Design review of the part built by this model. Coordinates are the model's own, in mm. Round coordinates to 2 decimals unless told otherwise and drop trailing zeros. Order: outer loops, then holes, each group sorted by start corner. A loop starts at its lowest first (then second) coordinate and runs counter-clockwise, first axis right, second up. Notation, with made-up numbers: M -9,-7 L 9,-7 A17 cw 9,7 Z; hole C 15.25,-4.75 d6. An arc over 180 degrees is marked long. Write each question's results on one line, items separated by ' | '. Start each with the question number.
Item 1: Wall thickness on line 1 (Y direction, x = 82.05, z = -3); line 2 (Z direction, x = 29.5, y = -16.5); line 3 (X direction, y = -26, z = -4): over which ranges is each line inside the solid? List them lowest first. Write a range as [from, to].
Item 2: Clearance check with flat-ended pins moving along their axes: pin 1 (6.5 mm diameter, centred on y = 0.5, z = -4, fed in from +X); pin 2 (3 mm diameter, centred on x = -39, y = -13, fed in from -Z); pin 3 (5 mm diameter, centred on x = -81, z = -5.5, fed in from -Y); pin 4 (1.2 mm diameter, centred on y = 5, z = 2.5, fed in from +X). State where each tip first meets the part, or that it passes through.
Item 3: Take a section at B-B, the plane x = 38. Write out the cut boundary in (y, z).
Item 4: Take a section at A-A, the plane y = 0. Write out the cut boundary in (x, z), plus the area to 3 significant figures.
Item 5: Take a section at C-C, the plane y = 8. Write out the cut boundary in (x, z), plus the area to 3 significant figures.
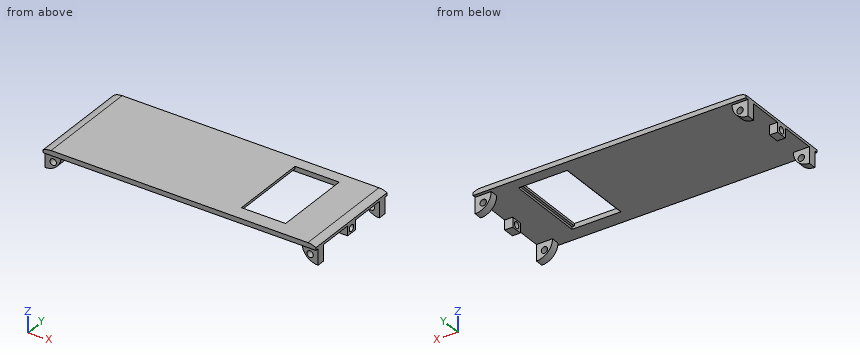
```python
from build123d import *

# Parameters (mm, degrees)
SKIZZE1_W                                  = 180
SKIZZE1_H                                  = 65
AUFSATZ_LINEAR_AUSTRAGEN1_DEPTH            = 3
SKIZZE3_W                                  = 5
SKIZZE3_H                                  = 7
AUFSATZ_LINEAR_AUSTRAGEN2_DEPTH            = 6
F_4_0_4_DURCHMESSER_BOHRUNG1_D             = 4
SCHNITT_LINEAR_AUSTRAGEN1_DEPTH            = 112.180034179
SKIZZE7_W                                  = 27.5
SKIZZE7_H                                  = 49
SCHNITT_LINEAR_AUSTRAGEN2_DEPTH            = 92.445338864
SKIZZE8_W                                  = 10
SKIZZE8_H                                  = 5
AUFSATZ_LINEAR_AUSTRAGEN3_DEPTH            = 10
SPIEGELN1_AT_THE_SECOND_PLANE_COPY_1_SKE_W = 10
SPIEGELN1_AT_THE_SECOND_PLANE_COPY_1_SKE_H = 5
SPIEGELN1_AT_THE_SECOND_PLANE_COPY_1_DEPTH = 10
VERRUNDUNG1_R                              = 10
F_4_0_4_DURCHMESSER_BOHRUNG2_D             = 4
F_4_0_4_DURCHMESSER_BOHRUNG2_DEPTH         = 5
F_4_0_4_DURCHMESSER_BOHRUNG3_D             = 4
F_4_0_4_DURCHMESSER_BOHRUNG3_DEPTH         = 5
SKIZZE13_W                                 = 30.5
SKIZZE13_H                                 = 49
SCHNITT_LINEAR_AUSTRAGEN4_DEPTH            = 1.5


with BuildPart() as part:
    # Skizze1 → Aufsatz-Linear austragen1 (new body)
    with BuildSketch(Plane.XY):
        Rectangle(SKIZZE1_W, SKIZZE1_H)
    extrude(amount=AUFSATZ_LINEAR_AUSTRAGEN1_DEPTH)

    # Skizze3 → Aufsatz-Linear austragen2 (add)
    with BuildSketch(Plane(origin=(0, 0, 0), x_dir=(-1, 0, 0), z_dir=(0, 0, -1))):
        with Locations((-82.5, 0)):
            Rectangle(SKIZZE3_W, SKIZZE3_H)
        with Locations((82.5, 0)):
            Rectangle(SKIZZE3_W, SKIZZE3_H)
    extrude(amount=AUFSATZ_LINEAR_AUSTRAGEN2_DEPTH)

    # Ø4.0 (4) Durchmesser Bohrung1 (through all)
    with Locations(Plane.ZY.offset(85)):
        with Locations((-3, 0)):
            Hole(F_4_0_4_DURCHMESSER_BOHRUNG1_D / 2)

    # Skizze6 → Schnitt-Linear austragen1 (cut, through all)
    with BuildSketch(Plane(origin=(0, 32.5, 0), x_dir=(1, 0, 0), z_dir=(0, 1, 0))):
        with BuildLine():
            Line((-80, -3), (-90, -3))
            Line((-90, -3), (-90, 0))
            Line((-90, 0), (-85, 0))
            Line((-85, 0), (-85, -1.660254038))
            ThreePointArc((-85, -1.660254038), (-82.588190451, -2.659258263), (-80, -3))
        make_face()
        with BuildLine():
            Line((80, -3), (90, -3))
            Line((90, -3), (90, 0))
            Line((90, 0), (85, 0))
            Line((85, 0), (85, -1.660254038))
            ThreePointArc((85, -1.660254038), (82.588190451, -2.659258263), (80, -3))
        make_face()
    extrude(amount=-SCHNITT_LINEAR_AUSTRAGEN1_DEPTH, mode=Mode.SUBTRACT)

    # Skizze7 → Schnitt-Linear austragen2 (cut, through all)
    with BuildSketch(Plane.XY.offset(3)):
        with Locations((46.25, 1)):
            Rectangle(SKIZZE7_W, SKIZZE7_H)
    extrude(amount=-SCHNITT_LINEAR_AUSTRAGEN2_DEPTH, mode=Mode.SUBTRACT)

    # Skizze8 → Aufsatz-Linear austragen3 (add)
    with BuildSketch(Plane(origin=(0, 0, 0), x_dir=(-1, 0, 0), z_dir=(0, 0, -1))):
        with Locations((-80, 28)):
            Rectangle(SKIZZE8_W, SKIZZE8_H)
    aufsatz_linear_austragen3 = extrude(amount=AUFSATZ_LINEAR_AUSTRAGEN3_DEPTH)

    # Spiegeln1: Aufsatz-Linear austragen3 across plane
    add(aufsatz_linear_austragen3.mirror(Plane(origin=(0, 0, 0), x_dir=(0, 0, 1), z_dir=(1, 0, 0))))

    # Spiegeln1 at the second plane: Aufsatz-Linear austragen3 across plane
    add(aufsatz_linear_austragen3.mirror(Plane.ZX))

    # Spiegeln1 at the second plane copy 1 ske → Spiegeln1 at the second plane copy 1 (add)
    with BuildSketch(Plane(origin=(0, 0, 0), x_dir=(1, 0, 0), z_dir=(0, 0, -1))):
        with Locations((-80, 28)):
            Rectangle(SPIEGELN1_AT_THE_SECOND_PLANE_COPY_1_SKE_W, SPIEGELN1_AT_THE_SECOND_PLANE_COPY_1_SKE_H)
    extrude(amount=SPIEGELN1_AT_THE_SECOND_PLANE_COPY_1_DEPTH)

    # Verrundung1
    verrundung1_edges = [part.edges().sort_by_distance(p)[0] for p in [
        (75, 28, -10),
        (75, -28, -10),
        (-75, 28, -10),
        (-75, -28, -10),
    ]]
    fillet(verrundung1_edges, radius=VERRUNDUNG1_R - 0.0001)  # a hair under: the kernel refuses the full size

    # Ø4.0 (4) Durchmesser Bohrung2
    with Locations(Plane(origin=(0, 30.5, 0), x_dir=(1, 0, 0), z_dir=(0, 1, 0))):
        with Locations((-80, 5), (80, 5)):
            Hole(F_4_0_4_DURCHMESSER_BOHRUNG2_D / 2, depth=F_4_0_4_DURCHMESSER_BOHRUNG2_DEPTH)

    # Ø4.0 (4) Durchmesser Bohrung3
    with Locations(Plane(origin=(0, -30.5, 0), x_dir=(-1, 0, 0), z_dir=(0, -1, 0))):
        with Locations((-80, 5), (80, 5)):
            Hole(F_4_0_4_DURCHMESSER_BOHRUNG3_D / 2, depth=F_4_0_4_DURCHMESSER_BOHRUNG3_DEPTH)

    # Skizze13 → Schnitt-Linear austragen4 (cut)
    with BuildSketch(Plane(origin=(0, 0, 0), x_dir=(-1, 0, 0), z_dir=(0, 0, -1))):
        with Locations((-46.25, 1)):
            Rectangle(SKIZZE13_W, SKIZZE13_H)
    extrude(amount=-SCHNITT_LINEAR_AUSTRAGEN4_DEPTH, mode=Mode.SUBTRACT)


solid = part.part
```
Results list:
1) line 1: [-30.5, -25.5], [-3.5, -2], [2, 3.5], [25.5, 30.5] | line 2: [0, 3] | line 3: [-85, -81.73], [-78.27, -75.83], [75.83, 78.27], [81.73, 85]
2) pin 1: x = 85 | pin 2: z = 0 | pin 3: y = -30.5 | pin 4: x = 84.56
3) outline: M -32.5,0 L -23.5,0 L -23.5,3 L -32.5,3 Z; M 25.5,0 L 32.5,0 L 32.5,3 L 25.5,3 Z
4) outline: M -85,-6 L -80,-6 L -80,-5 L -85,-5 Z; M -85,-1 L -80,-1 L -80,0 L 31,0 L 31,1.5 L 32.5,1.5 L 32.5,3 L -80,3 A10 ccw -85,1.66 Z; M 60,1.5 L 61.5,1.5 L 61.5,0 L 80,0 L 80,-1 L 85,-1 L 85,1.66 A10 ccw 80,3 L 60,3 Z; M 80,-6 L 85,-6 L 85,-5 L 80,-5 Z | area: 439 mm²
5) outline: M -85,0 L 31,0 L 31,1.5 L 32.5,1.5 L 32.5,3 L -80,3 A10 ccw -85,1.66 Z; M 60,1.5 L 61.5,1.5 L 61.5,0 L 85,0 L 85,1.66 A10 ccw 80,3 L 60,3 Z | area: 419 mm²
